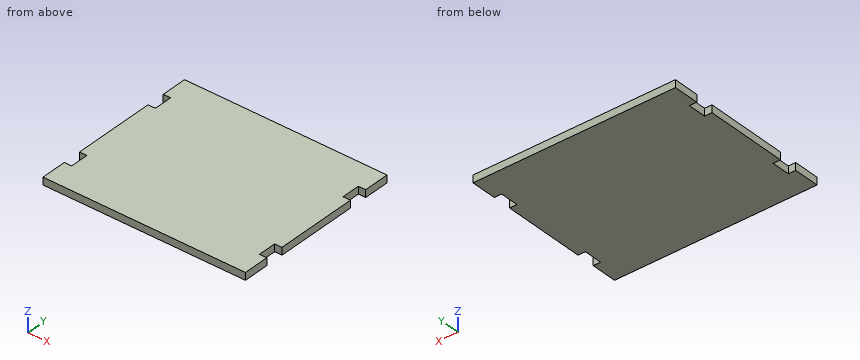
Autodesk Inventor part; units mm, degrees
ref_plane "YZ Plane" through (0, 0, 0) normal (1, 0, 0) x (0, 1, 0)
ref_plane "XZ Plane" through (0, 0, 0) normal (0, 1, 0) x (-1, 0, 0)
ref_plane "XY Plane" through (0, 0, 0) normal (0, 0, 1) x (1, 0, 0)
sketch "Sketch1" plane through (0, 0, 0) normal (0, 0, 1) x (1, 0, 0)
  line L0 (0, -24) -> (0, -14)
  line L1 (4, -14) -> (4, -24)
  line L2 (0, -79) -> (0, -69)
  line L3 (4, -69) -> (4, -79)
  line L4 (0, -69) -> (4, -69)
  line L5 (0, -79) -> (4, -79)
  line L6 (106, -79) -> (106, -69)
  line L7 (110, -69) -> (110, -79)
  line L8 (110, -14) -> (106, -14)
  line L9 (110, -24) -> (106, -24)
  line L10 (106, -24) -> (106, -14)
  line L11 (110, -14) -> (110, -24)
  line L12 (0, 0) -> (110, 0)
  line L13 (110, 0) -> (110, -93)
  line L14 (110, -93) -> (0, -93)
  line L15 (0, -93) -> (0, 0)
  line L16 (4, -14) -> (0, -14)
  line L17 (0, -14) -> (0, -24)
  line L18 (0, -24) -> (4, -24)
  line L19 (4, -24) -> (4, -14)
  line L20 (106, -69) -> (110, -69)
  line L21 (110, -69) -> (110, -79)
  line L22 (110, -79) -> (106, -79)
  line L23 (106, -79) -> (106, -69)
extrude "Extrusion1" add sketch "Sketch1" along normal blind 4 contours L18 L1 L16 L15 L12 L13 L8 L10 L9 L20 L6 L22 L14 L5 L3 L4
properties part number "TAPA_CAJA"
Geometry: final body of the model. Coordinates: model frame, mm. Round coordinates to 2 decimals unless told otherwise and drop trailing zeros. Order: outer loops, then holes, each group sorted by start corner. A loop starts at its lowest first (then second) coordinate and runs counter-clockwise, first axis right, second up. Notation, with made-up numbers: (-19, 38) -> (-4, 38) arc R26 ccw to (-4, 72) -> close; hole circle Ø4 at (15.5, -14.75). An arc over 180 degrees is marked (long way). Put each result on its own line as item: value. Start each with the question number.
Q1. Line query: probe 1 along X at (y, z) = (-18, 2.1). Output: solid intervals per line, ascending.
Q2. First-contact query: pin 1 (1.2 mm diameter, centred on y = -75.5, z = 2, fed in from +X); pin 2 (2 mm diameter, centred on y = -76.5, z = 1.5, fed in from -X). Flat tips, straight axial feed; report the tip coordinate or a pass-through.
Q3. Section A-A on z = 1.85. Return the cut outline in (x, y).
Q4. Section B-B on y = -73. Return the cut outline in (x, z), and give its area (3 significant figures).
Ans:
1. probe 1: x = 4 to 106
2. pin 1: stops at x = 106
2. pin 2: stops at x = 4
3. outline: (0, -93) -> (110, -93) -> (110, -79) -> (106, -79) -> (106, -69) -> (110, -69) -> (110, -24) -> (106, -24) -> (106, -14) -> (110, -14) -> (110, 0) -> (0, 0) -> (0, -14) -> (4, -14) -> (4, -24) -> (0, -24) -> (0, -69) -> (4, -69) -> (4, -79) -> (0, -79) -> close
4. outline: (4, 0) -> (106, 0) -> (106, 4) -> (4, 4) -> close
4. area: 408 mm2
